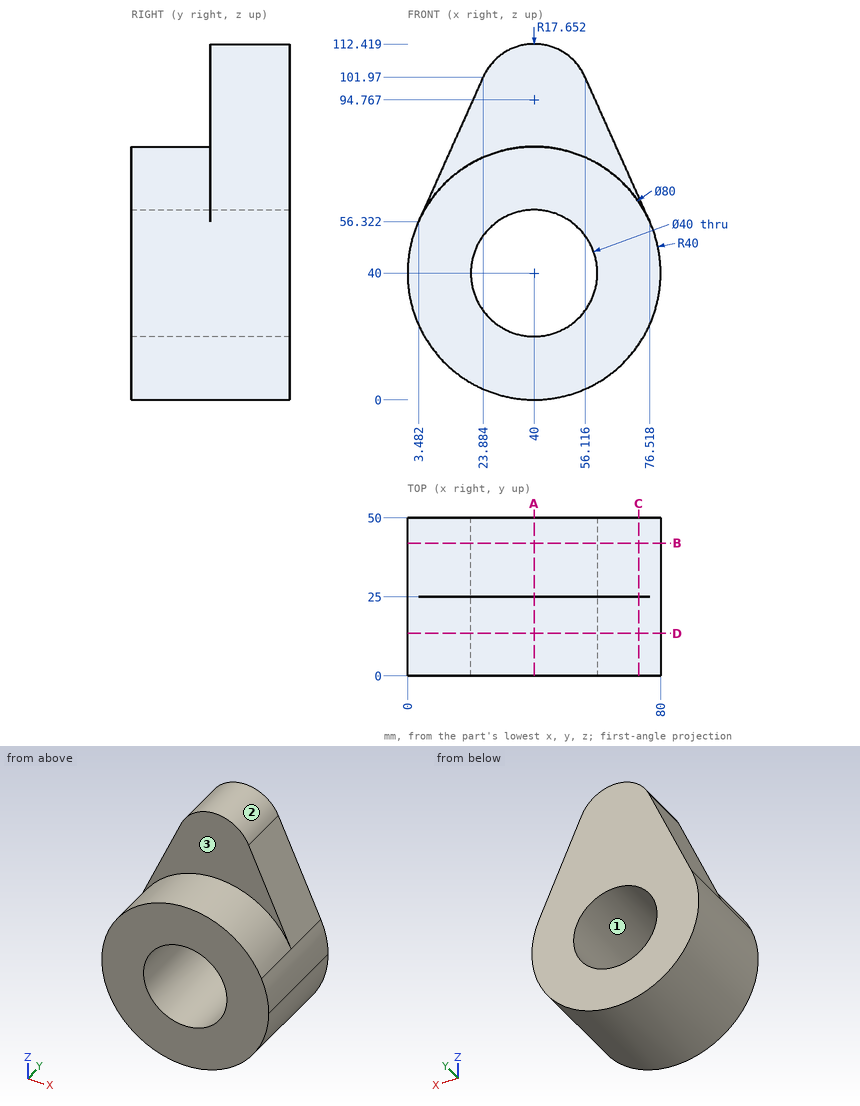
The drawing under review shows one solid part. Ordinate dimensions are in mm from its lowest x, y, z. Round coordinates to 2 decimals unless told otherwise and drop trailing zeros. Loops run counter-clockwise (first coordinate to the right, second up) from the corner with the lowest first, then second, coordinate; pieces in that order, holes last. Notation, with made-up numbers: (35.25, 89.25) -> (61.25, 89.25) arc R25 cw to (61.25, 112.25) -> close; hole circle Ø1 at (57, 71.5). An arc over 180 degrees is marked (long way). One line per question, with ' | ' between items. Start each with the question number.
Item 1: Draft analysis for pull direction Z (two halves, no side actions). For the marked faces 1, 2 and 3, state which applies: +Z half, -Z half, draft (parallel to the pull), parting line (faces both ways), or undercut.
Item 2: Add section C-C, the plane x = 73. Write out the cut boundary in (y, z) (1 decimal), then the cut area to 3 significant figures.
Item 3: Wall thickness on line 1 along X through (y, z) = (14.5, 40); line 2 along Z through (x, y) = (40, 34): over which ranges is each line inside the solid? List them lowest first. Write a range as [from, to].
Item 4: Add section D-D, the plane y = 13.5. Write out the cut boundary in (x, z), then the cut area to 3 significant figures.
Item 5: Add section A-A, the plane x = 40. Write out the cut boundary in (y, z), then the cut area to 3 significant figures.
Item 6: For pin 1 (1 mm diameter, centred on x = 12.5, y = 21, fed in from +Z); pin 2 (3 mm diameter, centred on x = 52, y = 44.5, fed in from +Z); pin 3 (5 mm diameter, centred on y = 33, z = 68.5, fed in from +X), all flat-tipped, find the tip position at first contact; note any pin that passes through.
Item 7: Add section B-B, the plane y = 42. Write out the cut boundary in (x, z) (1 decimal).
Return value:
1) face 1: undercut | face 2: +Z half | face 3: draft
2) outline: (0, 17.4) -> (50, 17.4) -> (50, 64.2) -> (25, 64.2) -> (25, 62.6) -> (0, 62.6) -> close | area: 2,300 mm2
3) line 1: x = [0, 20], [60, 80] | line 2: z = [0, 20], [60, 112.42]
4) outline: (76.52, 56.32) arc R40 ccw (long way) to (80, 40) arc R40 ccw to start; hole circle Ø40 at (40, 40) | area: 3,770 mm2
5) outline: (0, 0) -> (50, 0) -> (50, 20) -> (0, 20) -> close; (0, 60) -> (50, 60) -> (50, 112.42) -> (25, 112.42) -> (25, 80) -> (0, 80) -> close | area: 2,810 mm2
6) pin 1: stops at z = 69.51 | pin 2: stops at z = 108.96 | pin 3: stops at x = 72.19
7) outline: (3.5, 56.3) arc R40 ccw (long way) to (80, 40) arc R40 ccw to (76.5, 56.3) -> (56.1, 102) arc R17.7 ccw to (23.9, 102) -> close; hole circle Ø40 at (40, 40)
